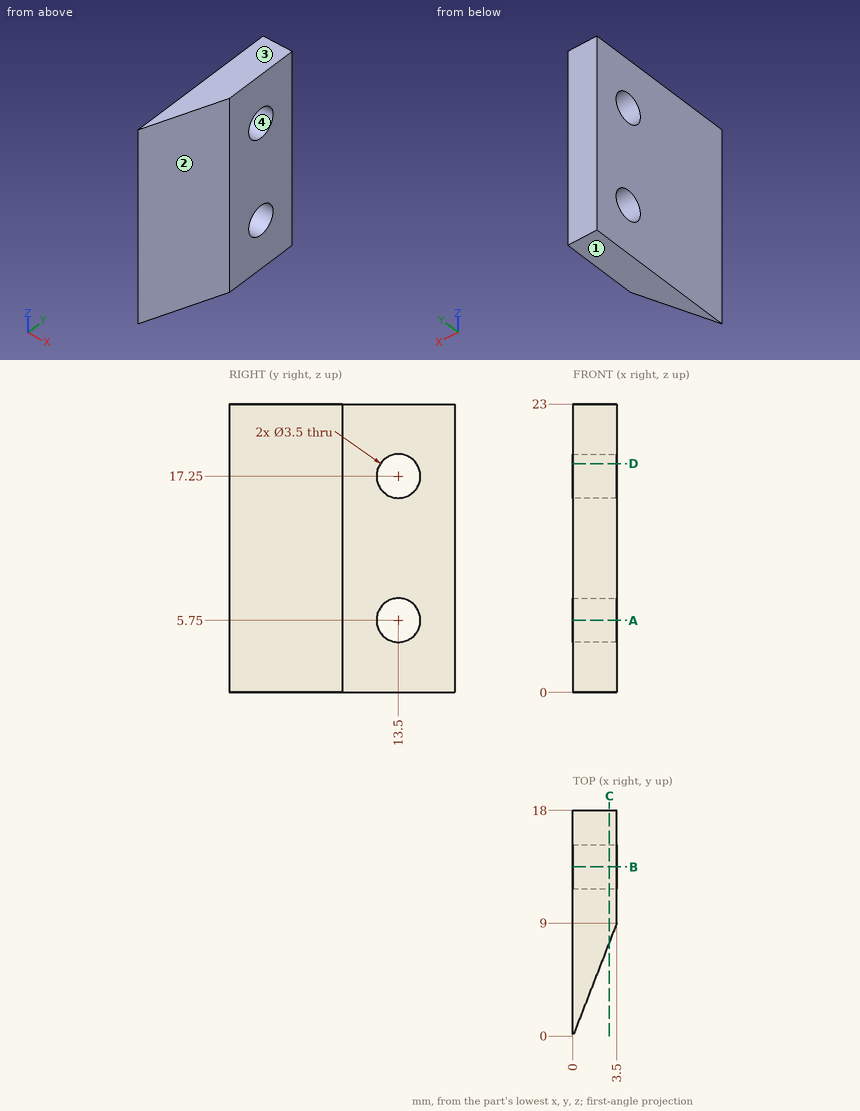
Drawing for the job (mm, zero at the part's lowest x, y, z). Coordinates: 2 decimals unless noted, no trailing zeros. Order: outer loops, then holes, each group sorted by start corner. A loop starts at its lowest first (then second) coordinate and runs counter-clockwise, first axis right, second up. Notation, with made-up numbers: (51, -22) - (105, -22) arc R11 ccw to (105, -1) - close; hole circle Ø11 at (21, 50.5). An arc over 180 degrees is marked (long way). Use a Markdown table: item, result. Add a question column.
(1) Saw through at C-C (x = 2.9). Give the cut face in (y, z).
(2) Pull direction Z, two halves, no side cores. Call the marked faces 1, 2, 3 and 4: +Z half, -Z half, draft (parallel to the pull), parting line (faces both ways), or undercut.
(3) Saw through at D-D (z = 18.25). Give the cut face in (x, y), then the cut area to 3 significant figures.
(4) Saw through at A-A (z = 5.75). Give the cut face in (x, y).
(5) Saw through at B-B (y = 13.5). Give the cut face in (x, z).
(6) Drill centre lines: line 1 along Z through (x, y) = (1.65, 13); line 2 along X through (y, z) = (4.75, 5.75); line 3 along X through (y, z) = (3.25, 12.5). Where is each one in solid material? Low to high. Write a range as [from, to].
Solved:
| question | item | result |
|---|---|---|
| 1 | outline | (7.46, 0) - (18, 0) - (18, 23) - (7.46, 23) - close; hole circle Ø3.5 at (13.5, 5.75); hole circle Ø3.5 at (13.5, 17.25) |
| 2 | face 1 | -Z half |
| 2 | face 2 | draft |
| 2 | face 3 | +Z half |
| 2 | face 4 | undercut |
| 3 | outline | (0, 0) - (3.5, 9) - (3.5, 12.06) - (0, 12.06) - close; (0, 14.94) - (3.5, 14.94) - (3.5, 18) - (0, 18) - close |
| 3 | area | 37.2 mm² |
| 4 | outline | (0, 0) - (3.5, 9) - (3.5, 11.75) - (0, 11.75) - close; (0, 15.25) - (3.5, 15.25) - (3.5, 18) - (0, 18) - close |
| 5 | outline | (0, 0) - (3.5, 0) - (3.5, 4) - (0, 4) - close; (0, 7.5) - (3.5, 7.5) - (3.5, 15.5) - (0, 15.5) - close; (0, 19) - (3.5, 19) - (3.5, 23) - (0, 23) - close |
| 6 | line 1 | z = [0, 4.07], [7.43, 15.57], [18.93, 23] |
| 6 | line 2 | x = [0, 1.85] |
| 6 | line 3 | x = [0, 1.26] |
